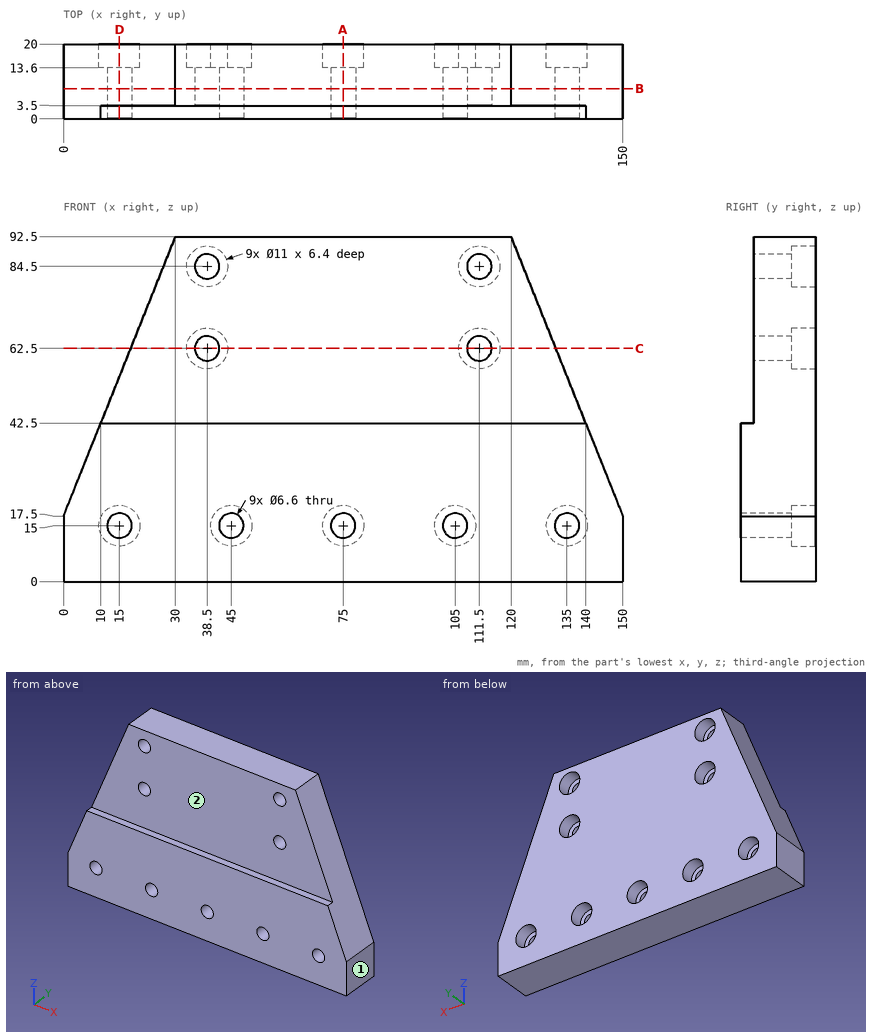
Geometry: see drawing. Coordinates: mm, zero at the bounding-box minimum. A direction names the side the tool comes from. Round coordinates to 2 decimals unless told otherwise and drop trailing zeros. Loops run counter-clockwise (first coordinate to the right, second up) from the corner with the lowest first, then second, coordinate; pieces in that order, holes last. Notation, with made-up numbers: (60, 20.5) -> (75, 20.5) arc R38 cw to (75, 58.5) -> close; hole circle Ø2 at (-10, -2). An arc over 180 degrees is marked (long way). Write each question's results on one line, items separated by ' | '.
1. Section A-A (x = 75). Return loops of the section in (y, z), and give its area (3 significant figures).
Geometry results:
outline: (0, 0) -> (20, 0) -> (20, 9.5) -> (13.6, 9.5) -> (13.6, 11.7) -> (0, 11.7) -> close; (0, 18.3) -> (13.6, 18.3) -> (13.6, 20.5) -> (20, 20.5) -> (20, 92.5) -> (3.5, 92.5) -> (3.5, 42.5) -> (0, 42.5) -> close | area: 1,510 mm2
2. Set-up query: the marked faces 1 and 2. Return all of +Z, -Z, +X, -X, +Y, -Y with unobstructed straight access to the full face (end or side cutting, diameter ignored); none if empty.
Geometry results:
face 1: +Z, -Z, +X, +Y, -Y | face 2: +Z, +X, -X, -Y
3. First-contact query: P1, Ø8, axis at x = 64, z = 51.5, coming from the -Y side; P2, Ø1, axis at x = 97.5, y = 2, coming from the +Z side; P3, Ø12, axis at y = 4, z = 58.5, coming from the +X side. Flat tips, straight axial feed; report the tip coordinate or a pass-through.
Geometry results:
P1: y = 3.5 | P2: z = 42.5 | P3: x = 136
4. Ray query, line 1 (X direction, y = 16.5, z = 15); line 2 (Z direction, x = 111.5, y = 6); line 3 (X direction, y = 4.25, z = 15). Return the intervals inside material, ascending. Write a range as from..to.
Geometry results:
line 1: 0..9.5, 20.5..39.5, 50.5..69.5, 80.5..99.5, 110.5..129.5, 140.5..150 | line 2: 0..59.2, 65.8..81.2, 87.8..92.5 | line 3: 0..11.7, 18.3..41.7, 48.3..71.7, 78.3..101.7, 108.3..131.7, 138.3..150
5. Section B-B (y = 8). State how many separate pieces and enclosed holes the cut face has, and give its area (3 significant figures).
Geometry results:
separate pieces: 1 | enclosed holes: 9 | area: 11,300 mm2
6. Section D-D (x = 15). Return loops of the section in (y, z), and give its area (3 significant figures).
Geometry results:
outline: (0, 0) -> (20, 0) -> (20, 9.5) -> (13.6, 9.5) -> (13.6, 11.7) -> (0, 11.7) -> close; (0, 18.3) -> (13.6, 18.3) -> (13.6, 20.5) -> (20, 20.5) -> (20, 55) -> (3.5, 55) -> (3.5, 42.5) -> (0, 42.5) -> close | area: 896 mm2
7. Section C-C (z = 62.5). Return loops of the section in (x, y), and give its area (3 significant figures).
Geometry results:
outline: (18, 3.5) -> (35.2, 3.5) -> (35.2, 13.6) -> (33, 13.6) -> (33, 20) -> (18, 20) -> close; (41.8, 3.5) -> (108.2, 3.5) -> (108.2, 13.6) -> (106, 13.6) -> (106, 20) -> (44, 20) -> (44, 13.6) -> (41.8, 13.6) -> close; (114.8, 3.5) -> (132, 3.5) -> (132, 20) -> (117, 20) -> (117, 13.6) -> (114.8, 13.6) -> close | area: 1,610 mm2
